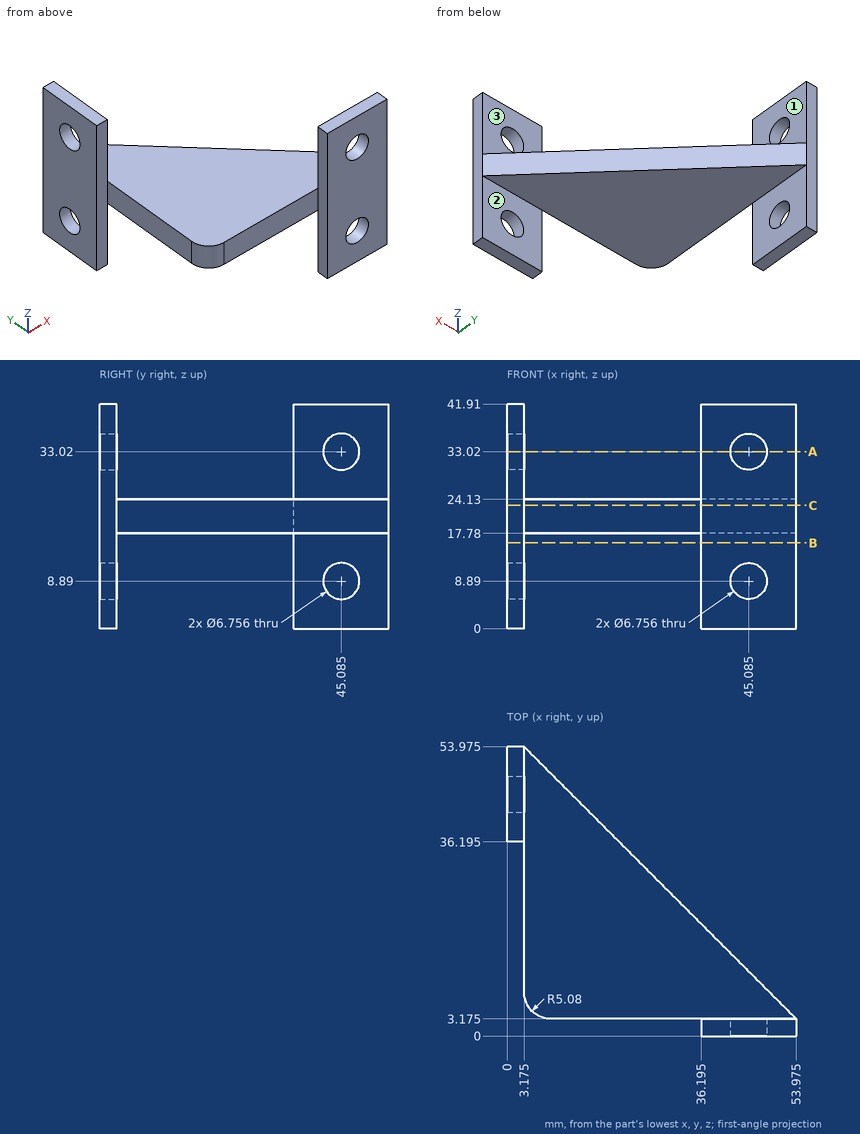
Can you work these out from the drawing? Everything is in mm from the part's minimum corner. A direction names the side the tool comes from. Round coordinates to 2 decimals unless told otherwise and drop trailing zeros. Loops run counter-clockwise (first coordinate to the right, second up) from the corner with the lowest first, then second, coordinate; pieces in that order, holes last. Notation, with made-up numbers: (34.5, -32) -> (74.5, -32) arc R19 ccw to (74.5, -10) -> close; hole circle Ø8 at (46, 79). An arc over 180 degrees is marked (long way). Answer in a Markdown table with one row per item.
Item 1: Suppose I cut it at C-C, the plane z = 23. List the corners of the cut face in (x, y) for me (1 decimal).
Answer block:
| item | result |
|---|---|
| outline | (0, 36.2) -> (3.2, 36.2) -> (3.2, 8.3) arc R5.1 ccw to (8.3, 3.2) -> (36.2, 3.2) -> (36.2, 0) -> (54, 0) -> (54, 3.2) -> (3.2, 54) -> (0, 54) -> close |
Item 2: On a 3-axis mill with a long thin cutter (end or side, diameter ignored), from which of +Z, -Z, +X, -X, +Y, -Y can I reach the whole of each face in a straight line? I mean the marked faces 1, 2 and 3. Say none if no direction works.
Answer block:
| item | result |
|---|---|
| face 1 | +Z, +X, +Y, -Y |
| face 2 | -Z, +X, -X, +Y |
| face 3 | +Z, +X, -X, +Y |
Item 3: If I drill on probe 1 along Y at (x, z) = (1.5, 33.02) (1 decimal); probe 2 along Z at (x, y) = (50, 5); probe 3 along X at (y, z) = (51, 29) (1 decimal), over which ranges is the centre line in solid material (lowest first)?
Answer block:
| item | result |
|---|---|
| probe 1 | 36.2 to 41.7, 48.5 to 54 |
| probe 2 | 17.78 to 24.13 |
| probe 3 | 0 to 3.2 |
Item 4: Will these pins go through, and if not, where does the flat tip stop? P1, Ø6, axis at x = 22.5, y = 28, coming from the -Z side; P2, Ø10, axis at x = 39, z = 14.5, coming from the +Y side (1 decimal); P3, Ø19.5, axis at y = 43.5, z = 34, coming from the +X side (3 decimals).
Answer block:
| item | result |
|---|---|
| P1 | z = 17.78 |
| P2 | y = 21.9 |
| P3 | x = 3.175 |
Item 5: Suppose I cut it at A-A, the plane z = 33.02. List the corners of the cut face in (x, y) for me (1 decimal).
Answer block:
| item | result |
|---|---|
| outline | (0, 36.2) -> (3.2, 36.2) -> (3.2, 41.7) -> (0, 41.7) -> close; (0, 48.5) -> (3.2, 48.5) -> (3.2, 54) -> (0, 54) -> close; (36.2, 0) -> (41.7, 0) -> (41.7, 3.2) -> (36.2, 3.2) -> close; (48.5, 0) -> (54, 0) -> (54, 3.2) -> (48.5, 3.2) -> close |
Item 6: Suppose I cut it at B-B, the plane z = 16. List the corners of the cut face in (x, y) for me (1 decimal).
Answer block:
| item | result |
|---|---|
| outline | (0, 36.2) -> (3.2, 36.2) -> (3.2, 54) -> (0, 54) -> close; (36.2, 0) -> (54, 0) -> (54, 3.2) -> (36.2, 3.2) -> close |
